```python
from build123d import *

# Parameters (mm, degrees)
SALIENTE_EXTRUIR1_DEPTH       = 15
SALIENTE_EXTRUIR1_DEPTH_BACK  = 15
SALIENTE_EXTRUIR3_DEPTH       = 10
SALIENTE_EXTRUIR3_DEPTH_BACK  = 10
SALIENTE_EXTRUIR9_DEPTH       = 5
SALIENTE_EXTRUIR9_DEPTH_BACK  = 25
CROQUIS4_R                    = 8.75
SALIENTE_EXTRUIR10_DEPTH      = 10
SALIENTE_EXTRUIR10_DEPTH_BACK = 10
CROQUIS5_R                    = 8.75
CROQUIS6_R                    = 13.287682
SALIENTE_EXTRUIR11_DEPTH      = 8
CROQUIS7_R                    = 15.287682
SALIENTE_EXTRUIR12_DEPTH      = 17
SALIENTE_EXTRUIR13_DEPTH      = 17
SALIENTE_EXTRUIR13_DEPTH_BACK = 17
CROQUIS9_R                    = 15.287682
SALIENTE_EXTRUIR14_DEPTH      = 2
SALIENTE_EXTRUIR14_DEPTH_BACK = 36
SALIENTE_EXTRUIR15_DEPTH      = 5
SALIENTE_EXTRUIR15_DEPTH_BACK = 35
CROQUIS11_W                   = 34.848077
CROQUIS11_H                   = 11.736482
CROQUIS12_R                   = 1.5
CORTAR_EXTRUIR1_DEPTH         = 35000
CROQUIS13_R                   = 1.5
CORTAR_EXTRUIR2_DEPTH         = 35000


with BuildPart() as part:
    # Croquis1 → Saliente-Extruir1 (new, two sides: drawn at the far end of the back side and taken through both)
    with BuildSketch(Plane(origin=(0, 0, 0), x_dir=(1, 0, 0), z_dir=(0, 1, 0)).offset(-SALIENTE_EXTRUIR1_DEPTH_BACK)):
        Polygon((0, 0), (0, 20), (-15.320889, 32.855752), (-25.168966, 21.11927), align=None)
    extrude(amount=SALIENTE_EXTRUIR1_DEPTH + SALIENTE_EXTRUIR1_DEPTH_BACK)

    # Croquis2 → Saliente-Extruir3 (add, two sides: drawn at the far end of the back side and taken through both)
    with BuildSketch(Plane(origin=(0, 0, 0), x_dir=(1, 0, 0), z_dir=(0, 1, 0)).offset(-SALIENTE_EXTRUIR3_DEPTH_BACK)):
        with BuildLine():
            Line((0, 0), (-13.405778, 11.248783))
            Line((-13.405778, 11.248783), (-19.190866, 4.354383))
            ThreePointArc((-19.190866, 4.354383), (-18.112369, -7.972897), (-5.785088, -6.8944))
            Line((-5.785088, -6.8944), (0, 0))
        make_face()
    extrude(amount=SALIENTE_EXTRUIR3_DEPTH + SALIENTE_EXTRUIR3_DEPTH_BACK)

    # Croquis4 → Saliente-Extruir9 (add, two sides: drawn at the far end of the back side and taken through both)
    with BuildSketch(Plane(origin=(0, 10, 0), x_dir=(1, 0, 0), z_dir=(0, 1, 0)).offset(-SALIENTE_EXTRUIR9_DEPTH_BACK)):
        with Locations(Location((-12.487977, -1.270008, 0), (0, 0, 270))):
            Circle(CROQUIS4_R)
    extrude(amount=SALIENTE_EXTRUIR9_DEPTH + SALIENTE_EXTRUIR9_DEPTH_BACK)

    # Croquis5 → Saliente-Extruir10 (add, two sides: drawn at the far end of the back side and taken through both)
    with BuildSketch(Plane(origin=(0, 0, 0), x_dir=(1, 0, 0), z_dir=(0, 1, 0)).offset(-SALIENTE_EXTRUIR10_DEPTH_BACK)):
        with Locations(Location((-12.487977, -1.270008, 0), (0, 0, 270))):
            Circle(CROQUIS5_R)
        with BuildLine():
            ThreePointArc((-5.785088, -6.8944), (-18.112369, -7.972897), (-19.190866, 4.354383))
            Line((-19.190866, 4.354383), (-24.975955, -2.540017))
            Line((-24.975955, -2.540017), (-11.570177, -13.7888))
            Line((-11.570177, -13.7888), (-5.785088, -6.8944))
        make_face()
    extrude(amount=SALIENTE_EXTRUIR10_DEPTH + SALIENTE_EXTRUIR10_DEPTH_BACK)

    # Croquis6 → Saliente-Extruir11 (add)
    with BuildSketch(Plane(origin=(-11.570177, 0, 13.7888), x_dir=(0.7660444431189747, 0, 0.6427876096865435), z_dir=(-0.6427876096865434, 0, 0.7660444431189746))):
        with Locations(Location((-8.75, 0, 0), (0, 0, 228.814075))):
            Circle(CROQUIS6_R)
    extrude(amount=SALIENTE_EXTRUIR11_DEPTH)

    # Croquis7 → Saliente-Extruir12 (add)
    with BuildSketch(Plane(origin=(-16.712478, 0, 19.917156), x_dir=(0.7660444431189747, 0, 0.6427876096865435), z_dir=(-0.6427876096865434, 0, 0.7660444431189746))):
        with Locations(Location((-8.75, 0, 0), (0, 0, 180))):
            Circle(CROQUIS7_R)
    extrude(amount=SALIENTE_EXTRUIR12_DEPTH)

    # Croquis9 → Saliente-Extruir13 (add, two sides: drawn at the far end of the back side and taken through both)
    with BuildSketch(Plane(origin=(0, 0, 0), x_dir=(1, 0, 0), z_dir=(0, 1, 0)).offset(-SALIENTE_EXTRUIR13_DEPTH_BACK)):
        with Locations(Location((-34.342756, -27.315519, 0), (0, 0, 270))):
            Circle(CROQUIS9_R)
    extrude(amount=SALIENTE_EXTRUIR13_DEPTH + SALIENTE_EXTRUIR13_DEPTH_BACK)

    # Croquis10 → Saliente-Extruir14 (add, two sides: drawn at the far end of the back side and taken through both)
    with BuildSketch(Plane(origin=(0, 17, 0), x_dir=(1, 0, 0), z_dir=(0, 1, 0)).offset(-SALIENTE_EXTRUIR14_DEPTH_BACK)):
        with BuildLine():
            Line((-49.630438, -27.315519), (-49.630438, -39.315519))
            Line((-49.630438, -39.315519), (-59.342756, -39.315519))
            Line((-59.342756, -39.315519), (-59.342756, -44.315519))
            Line((-59.342756, -44.315519), (-9.342756, -44.315519))
            Line((-9.342756, -44.315519), (-9.342756, -39.315519))
            Line((-9.342756, -39.315519), (-19.055074, -39.315519))
            Line((-19.055074, -39.315519), (-19.055074, -27.315519))
            ThreePointArc((-19.055074, -27.315519), (-34.342756, -12.027837), (-49.630438, -27.315519))
        make_face()
    extrude(amount=SALIENTE_EXTRUIR14_DEPTH + SALIENTE_EXTRUIR14_DEPTH_BACK)

    # Croquis11 → Saliente-Extruir15 (add, two sides: drawn at the far end of the back side and taken through both)
    with BuildSketch(Plane(origin=(0, 15, 0), x_dir=(1, 0, 0), z_dir=(0, 1, 0)).offset(-SALIENTE_EXTRUIR15_DEPTH_BACK)):
        with Locations((-12.744927, 26.987511)):
            Rectangle(CROQUIS11_W, CROQUIS11_H)
    extrude(amount=SALIENTE_EXTRUIR15_DEPTH + SALIENTE_EXTRUIR15_DEPTH_BACK)

    # Croquis12 → Cortar-Extruir1 (cut)
    with BuildSketch(Plane.XY.offset(-21.11927)):
        with Locations((-0.320889, 17)):
            Circle(CROQUIS12_R)
        with Locations((-25.320889, 17)):
            Circle(CROQUIS12_R)
        with Locations((-25.320889, -17)):
            Circle(CROQUIS12_R)
        with Locations((-0.320889, -17)):
            Circle(CROQUIS12_R)
    extrude(amount=-CORTAR_EXTRUIR1_DEPTH, mode=Mode.SUBTRACT)

    # Croquis13 → Cortar-Extruir2 (cut)
    with BuildSketch(Plane(origin=(0, 0, 39.315519), x_dir=(-1, 0, 0), z_dir=(0, 0, -1))):
        with Locations((54.342756, 14)):
            Circle(CROQUIS13_R)
        with Locations((54.342756, -14)):
            Circle(CROQUIS13_R)
        with Locations((14.342756, 14)):
            Circle(CROQUIS13_R)
        with Locations((14.342756, -14)):
            Circle(CROQUIS13_R)
    extrude(amount=-CORTAR_EXTRUIR2_DEPTH, mode=Mode.SUBTRACT)


solid = part.part
```
Read the model definition and answer for the solid it produces. Units are mm, in the model's axes. A direction names the side the tool comes from. Round coordinates to 2 decimals unless told otherwise and drop trailing zeros. Write each loop counter-clockwise with the first axis right and the second up, starting at its lowest first coordinate (ties: lowest second). Pieces come first, ordered by that corner, then holes. Notation, with made-up numbers: (-11.5, 73) - (15.5, 73) arc R24 ccw to (15.5, 99) - close; hole circle Ø6 at (-19, -35.75). An arc over 180 degrees is marked (long way). One line per item, written item: value.
Q1. For a pull along Z with two mould halves and no side action, classify faces 4 (the cylindrical face through (-3.812, -12.535, 0.131)), 5 (the flat face through (-54, 0, 39.316)), 6 (the flat face through (-35, 0, 44.316)), 7 (the flat face through (-9.343, 0, 42)) as pulls with the +Z half, pulls with the -Z half, needs draft (parallel to the pull), parting line crosses it, or undercut.
The answers:
face 4: undercut
face 5: pulls with the -Z half
face 6: pulls with the +Z half
face 7: needs draft
Q2. Each of these flat-tipped pins is pushed along its axis until it touches: P1, Ø6, axis at y = 2, z = -9.5, coming from the +X side; P2, Ø2.5, axis at x = -25.32, y = -17, coming from the -Z side; P3, Ø9, axis at x = -11, z = 1.5, coming from the +Y side. Where does it stop, or does it pass through?
The answers:
P1: stops at x = 0
P2: stops at z = 14.15
P3: stops at y = 15
Q3. Straight lines are drawn through the part: line 1 (Z direction, x = -19, y = -9.5); line 2 (Z direction, x = -56, y = -13); line 3 (X direction, y = -10, z = 32.5). For each, find the intervals that lie inside material, in ascending order. Write a range as from..to.
The answers:
line 1: z = -32.86..-15.94, -4.58..27.66, 39.32..44.32
line 2: z = 39.32..44.32
line 3: x = -49.63..-19.06
Q4. Which of the six approach directions +Z, -Z, +X, -X, +Y, -Y give full straight-line access (tool end or side, diameter ignored) to faces 1 (the flat face through (-5.4, 10, -4.2)), 2 (the cylindrical face through (-26.43, 18.01, -26.91)), 3 (the cylindrical face through (-12.844, 14.066, 41.781))?
The answers:
face 1: +Y
face 2: -Z
face 3: +Z
Q5. Find section A-A (z = -22). Determine the outline of the cut face in (x, y).
The answers:
outline: (-30.17, -20) - (4.68, -20) - (4.68, 20) - (-30.17, 20) - close; hole circle Ø3 at (-25.32, -17); hole circle Ø3 at (-25.32, 17); hole circle Ø3 at (-0.32, -17); hole circle Ø3 at (-0.32, 17)
Q6. Find section C-C (y = -8). Determine the outline of the cut face in (x, z).
The answers:
outline: (-59.34, 39.32) - (-49.63, 39.32) - (-49.63, 27.32) arc R15.29 ccw to (-39.18, 12.81) - (-33.39, 5.92) - (-31.54, 7.47) - (-26.4, 1.34) - (-24.98, 2.54) - (-13.41, -11.25) - (-25.17, -21.12) - (-30.17, -21.12) - (-30.17, -32.86) - (4.68, -32.86) - (4.68, -21.12) - (-1.33, -21.12) - (0, -20) - (0, 0) - (-11.57, 13.79) - (-10.15, 14.98) - (-15.29, 21.11) - (-13.44, 22.67) - (-19.06, 29.36) - (-19.06, 39.32) - (-9.34, 39.32) - (-9.34, 44.32) - (-59.34, 44.32) - close
